Part model, mm, in its own coordinate system. Face numbers are marked on the shaded views. A direction names the side the tool comes from. Round coordinates to 2 decimals unless told otherwise and drop trailing zeros. Loops run counter-clockwise (first coordinate to the right, second up) from the corner with the lowest first, then second, coordinate; pieces in that order, holes last.
1) Band-saw the part on C-C, the plane x = 5.25. Write the cut outline in (y, z), then the cut area to 3 significant figures.
2) Band-saw the part on D-D, the plane x = 2.75. Write the cut outline in (y, z), then the cut area to 3 significant figures.
3) Band-saw the part on A-A, the plane y = 0. Write the cut outline in (x, z), then the cut area to 3 significant figures.
4) 3-axis set-ups, long thin cutter, end or side, ignore diameter. For the marked faces 4 and 5: which of +Z, -Z, +X, -X, +Y, -Y reach the whole face in a straight line?
5) Mould opens along Z. For the marked faces 1, 2 and 3 say: +Z half, -Z half, draft (parallel to the pull), parting line (faces both ways), or undercut.
6) Drop flat-ended pins along their axis: P1, Ø3, axis at x = 3.5, y = -2, coming from the -Z side; P2, Ø4, axis at x = 1, z = -1, coming from the +Y side; P3, Ø1, axis at x = 3, z = -2.5, coming from the +Y side. Give the stop position or say it passes through.
7) Probe line 1 (Z direction, x = 4.75, y = 0); line 2 (Z direction, x = 3.75, y = 0); line 3 (X direction, y = -3, z = 1.5). List the from-to ranges inside material, lowest first.
Autodesk Inventor part; units mm, degrees
ref_plane "YZ Plane" through (0, 0, 0) normal (1, 0, 0) x (0, 1, 0)
ref_plane "XZ Plane" through (0, 0, 0) normal (0, 1, 0) x (-1, 0, 0)
ref_plane "XY Plane" through (0, 0, 0) normal (0, 0, 1) x (1, 0, 0)
sketch "Sketch1" plane through (0, 0, 0) normal (0, 0, 1) x (1, 0, 0)
  line L0 (0, 0) -> (4, 0)
  line L1 (4, 0) -> (4, 3)
  line L2 (4, 3) -> (0, 3)
  line L3 (0, 3) -> (0, 0)
  line L4 (4, 0) -> (7, 0)
  line L5 (7, 0) -> (7, 5)
  line L6 (7, 5) -> (4, 5)
  line L7 (4, 5) -> (4, 0)
  dimension "d0" = 4
  dimension "d1" = 3
  dimension "d2" = 3
  dimension "d3" = 5
revolve "Revolution1" add sketch "Sketch1" angle 360 about axis through (0, 0, 0) along (1, 0, 0)
fillet "Fillet1" radius 0.1 1 edges at (4, -3, 0)
chamfer "Chamfer1" distance 0.5 angle 45 2 edges at (4, -5, 0) (0, -3, 0)
sketch "Sketch2" plane through (0, 0, 0) normal (-1, 0, 0) x (0, 0, 1)
  point P0 (0, 0)
  point P1 (0, 0)
hole "Hole1" at (0, 0, 0) direction (1, 0, 0) diameter 2.459 end through all
properties part number "Top_Shaft 1" material "Stainless Steel"
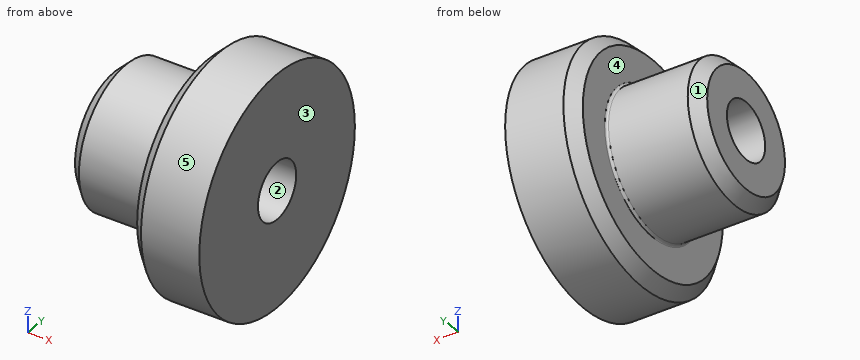
Reported:
1. outline: circle Ø10 at (0, 0); hole circle Ø2.46 at (0, 0)
1. area: 73.8 mm2
2. outline: circle Ø6 at (0, 0); hole circle Ø2.46 at (0, 0)
2. area: 23.5 mm2
3. outline: (0, -2.5) - (0.5, -3) - (3.9, -3) arc R0.1 cw to (4, -3.1) - (4, -4.5) - (4.5, -5) - (7, -5) - (7, -1.23) - (0, -1.23) - close; (0, 1.23) - (7, 1.23) - (7, 5) - (4.5, 5) - (4, 4.5) - (4, 3.1) arc R0.1 cw to (3.9, 3) - (0.5, 3) - (0, 2.5) - close
3. area: 36.3 mm2
4. face 4: -X
4. face 5: +X, -X
5. face 1: parting line
5. face 2: undercut
5. face 3: draft
6. P1: stops at z = -4.92
6. P2: stops at y = 3
6. P3: stops at y = 2.24
7. line 1: z = -5 to -1.23, 1.23 to 5
7. line 2: z = -3 to -1.23, 1.23 to 3
7. line 3: x = 4 to 7
